Here's how the part is built. I have some questions about the finished solid (model axes, mm). A direction names the side the tool comes from. Coordinates: 2 decimals unless noted, no trailing zeros. Write each loop counter-clockwise with the first axis right and the second up, starting at its lowest first coordinate (ties: lowest second). Pieces come first, ordered by that corner, then holes.
Item 1: If I drill on line 1 (X direction, y = 27, z = -11.75), over which ranges is the centre line in solid material (lowest first)?
Item 2: I'm going to push flat-ended pins straight in: pin 1 Ø17 at (x, y) = (18, -13) entering from +Z; pin 2 Ø1 at (y, z) = (7, -27) entering from +X; pin 3 Ø3 at (x, y) = (-12.5, 23.5) entering from -Z. Where does each tip first touch, or does it pass through?
Item 3: For faces 1 (the face through (23.7, -26.8, -26.7)), 2 (the face through (-15, 24, -2.25)), 3 (the face through (-3.2, 23.7, -26.7)), 4 (the face through (24, -15, -2.25)), 5 (the face through (-2.25, 24, -15)), which set-ups out of +Z, -Z, +X, -X, +Y, -Y let a thin tool reach every point of the face, with its end or its side?
Item 4: If we section it at A-A (y = 13.5): Please give me the cut outline in (x, z).
Item 5: If we section it at B-B (x = -16): Please give me the cut outline in (y, z), then the cut area to 3 significant figures.
Item 6: If we section it at C-C (z = -24.5): Please give me the cut outline in (x, y), then the cut area to 3 significant figures.
from build123d import *

# Parameters (mm, degrees)
SKETCH007_W     = 30
SKETCH007_H     = 30
PAD007_DEPTH    = 30
SKETCH008_W     = 25.5
SKETCH008_H     = 25.5
PAD008_DEPTH    = 50
CHAMFER002_SIZE = 2
SKETCH009_W     = 25.5
SKETCH009_H     = 25.5
PAD009_DEPTH    = 50
CHAMFER003_SIZE = 2


with BuildPart() as part:
    # Sketch007 → Pad007 (new body)
    with BuildSketch(Plane.XZ):
        with Locations((-15, -15)):
            Rectangle(SKETCH007_W, SKETCH007_H)
    extrude(amount=PAD007_DEPTH)

    # Sketch008 (on Face4 of Pad007) → Pad008 (join)
    with BuildSketch(Plane(origin=(0, 0, 0), x_dir=(0, 0, 1), z_dir=(1, 0, 0))):
        with Locations((-15, 15)):
            Rectangle(SKETCH008_W, SKETCH008_H)
    extrude(amount=PAD008_DEPTH)

    # Chamfer002
    chamfer002_edges = [part.edges().sort_by_distance(p)[0] for p in [
        (25, -27.75, -2.25),
        (25, -27.75, -27.75),
        (50, -27.75, -15),
        (50, -15, -2.25),
        (50, -15, -27.75),
        (50, -2.25, -15),
        (25, -2.25, -2.25),
        (25, -2.25, -27.75),
    ]]
    chamfer(chamfer002_edges, length=CHAMFER002_SIZE)

    # Sketch009 (on Face11 of Chamfer002) → Pad009 (join)
    with BuildSketch(Plane(origin=(0, 0, 0), x_dir=(1, 0, 0), z_dir=(0, 1, 0))):
        with Locations((-15, 15)):
            Rectangle(SKETCH009_W, SKETCH009_H)
    extrude(amount=PAD009_DEPTH)

    # Chamfer003
    chamfer003_edges = [part.edges().sort_by_distance(p)[0] for p in [
        (-2.25, 50, -15),
        (-15, 50, -27.75),
        (-27.75, 50, -15),
        (-15, 50, -2.25),
        (-27.75, 25, -2.25),
        (-27.75, 25, -27.75),
        (-2.25, 25, -2.25),
        (-2.25, 25, -27.75),
    ]]
    chamfer(chamfer003_edges, length=CHAMFER003_SIZE)


solid = part.part
Answer list:
1. line 1: x = -27.75 to -2.25
2. pin 1: stops at z = -2.25
2. pin 2: stops at x = -3
2. pin 3: stops at z = -27.75
3. face 1: -Z, +X, -Y
3. face 2: +Z, +X, -X, +Y
3. face 3: -Z, +X, +Y
3. face 4: +Z, +X, +Y, -Y
3. face 5: +Z, -Z, +X, +Y
4. outline: (-27.75, -25.75) - (-25.75, -27.75) - (-4.25, -27.75) - (-2.25, -25.75) - (-2.25, -4.25) - (-4.25, -2.25) - (-25.75, -2.25) - (-27.75, -4.25) - close
5. outline: (-30, -30) - (0, -30) - (0, -27.75) - (48, -27.75) - (50, -25.75) - (50, -4.25) - (48, -2.25) - (0, -2.25) - (0, 0) - (-30, 0) - close
5. area: 2,170 mm2
6. outline: (-30, -30) - (0, -30) - (0, -27.75) - (48, -27.75) - (50, -25.75) - (50, -4.25) - (48, -2.25) - (0, -2.25) - (0, 0) - (-2.25, 0) - (-2.25, 48) - (-4.25, 50) - (-25.75, 50) - (-27.75, 48) - (-27.75, 0) - (-30, 0) - close
6. area: 3,440 mm2
